For this review, take the finished solid that the model builds, in its own axes (mm). A direction names the side the tool comes from. Round coordinates to 2 decimals unless told otherwise and drop trailing zeros. Order: outer loops, then holes, each group sorted by start corner. A loop starts at its lowest first (then second) coordinate and runs counter-clockwise, first axis right, second up. Notation, with made-up numbers: (49, 26.5) - (62, 26.5) arc R20 cw to (62, 48.5) - close; hole circle Ø5 at (12, -28). An arc over 180 degrees is marked (long way). Write each question's results on one line, items separated by ' | '. Start each with the question number.
(1) Insertion check: pin 1 Ø4 at (x, y) = (4.5, -2.5) entering from +Z; pin 2 Ø4 at (x, y) = (15.5, 3) entering from +Z; pin 3 Ø10.5 at (x, z) = (0, 43.5) entering from +Y; pin 4 Ø6.5 at (y, z) = (-2, 13.5) entering from -X. Each pin has a flat end and moves straight along its axis. Give the tip position at first contact, or say it passes through.
(2) Take a section at C-C, the plane z = 43.5. Give the boundary of the cut face in (x, y).
(3) Take a section at D-D, the plane y = 5.75. Give the boundary of the cut face in (x, z).
(4) For L1, parallel to Z at x = 5.5, y = -0.75; L2, parallel to X at y = -3.5, z = 24.5; L3, parallel to Y at x = -9.4, z = 1.2, list the stretches that pass through material, from the lowest coordinate up. Write a range as from..to.
(5) Draft analysis for pull direction Y (two halves, no side actions). For faces 1 (the cylindrical face through (0, 0, 53)), 2 (the flat face through (0, 6.5, 22)), 3 (the cylindrical face through (8.66, 3.32, 1.97)), state which applies: pulls with the +Y half, pulls with the -Y half, needs draft (parallel to the pull), parting line crosses it, or undercut.
(6) For faces 4 (the flat face through (-3.5, 0, 19)), 5 (the flat face through (13, 0, 4)), 6 (the flat face through (0, 0, 0)), 7 (the cylindrical face through (-6.26, 1.3, 1.97)), 8 (the flat face through (20, 0, 2)), list the 3-axis set-ups (+Z, -Z, +X, -X, +Y, -Y) from which the entire face can be reached by the end or side of a thin tool; tool diameter is ignored.
(7) Take a section at A-A, the plane y = 0. Give the boundary of the cut face in (x, z).
(8) Take a section at B-B, the plane x = 0. Give the boundary of the cut face in (y, z), plus the area to 3 significant figures.
Autodesk Inventor part; units mm, degrees
ref_plane "工作平面3" through (-20, 0, 0) normal (0, 1, 0) x (1, 0, 0)
ref_plane "YZ Plane" through (0, 0, 0) normal (1, 0, 0) x (0, 1, 0)
ref_plane "XZ Plane" through (0, 0, 0) normal (0, 1, 0) x (-1, 0, 0)
sketch "草圖1" plane through (0, 0, 0) normal (0, 0, 1) x (1, 0, 0)
  line L0 (-20, 6.5) -> (20, 6.5)
  line L1 (20, 6.5) -> (20, -6.5)
  line L2 (20, -6.5) -> (-20, -6.5)
  line L3 (-20, -6.5) -> (-20, 6.5)
  line L4 (-20, 6.5) -> (20, -6.5) construction
  line L5 (20, 6.5) -> (-20, -6.5) construction
  circle A0 centre (-9.4, 0) radius 3.4
  circle A1 centre (9.4, 0) radius 3.4
  point P0 (0, 0)
  dimension "d0" = 40
  dimension "d1" = 13
  dimension "d2" = 6.8
  dimension "d3" = 6.8
extrude "擠出1" add sketch "草圖1" along normal blind 4
sketch "草圖3" plane through (0, 0, 4) normal (0, 0, 1) x (1, 0, 0)
  line L0 (3.5, -6.5) -> (-3.5, -6.5)
  line L1 (-3.5, -6.5) -> (-3.5, 6.5)
  line L2 (-3.5, 6.5) -> (3.5, 6.5)
  line L3 (3.5, 6.5) -> (3.5, -6.5)
  line L4 (3.5, -6.5) -> (-3.5, 6.5) construction
  line L5 (-3.5, -6.5) -> (3.5, 6.5) construction
  point P0 (0, 0)
  dimension "d8" = 7
  dimension "d9" = 13
extrude "擠出2" add sketch "草圖3" along normal blind 33
ref_plane "工作平面3" through (-20, 0, 0) normal (0, 1, 0) x (1, 0, 0)
sketch "草圖5" plane through (-20, 0, 0) normal (0, 1, 0) x (1, 0, 0)
  circle A0 centre (20, -43.5) radius 6.5
  circle A1 centre (20, -43.5) radius 9.5
  point P0 (20, 0)
  dimension "d22" = 13
  dimension "d23" = 19
extrude "擠出4" add sketch "草圖5" along normal mid plane 13
properties part number "T字形固定件v2"
Results below:
1) pin 1: stops at z = 52.67 | pin 2: stops at z = 4 | pin 3: passes through | pin 4: stops at x = -3.5
2) outline: (-9.5, -6.5) - (-6.5, -6.5) - (-6.5, 6.5) - (-9.5, 6.5) - close; (6.5, -6.5) - (9.5, -6.5) - (9.5, 6.5) - (6.5, 6.5) - close
3) outline: (-20, 0) - (20, 0) - (20, 4) - (3.5, 4) - (3.5, 34.67) arc R9.5 ccw (long way) to (-3.5, 34.67) - (-3.5, 4) - (-20, 4) - close; hole circle Ø13 at (0, 43.5)
4) L1: z = 0..4, 35.75..40.04, 46.96..51.25 | L2: x = -3.5..3.5 | L3: y = -6.5..-3.4, 3.4..6.5
5) face 1: needs draft | face 2: pulls with the +Y half | face 3: undercut
6) face 4: -X, +Y, -Y | face 5: +X, +Y, -Y | face 6: -Z, +X, -X, +Y, -Y | face 7: -Z | face 8: +Z, -Z, +X, +Y, -Y
7) outline: (-20, 0) - (-12.8, 0) - (-12.8, 4) - (-20, 4) - close; (-6, 0) - (6, 0) - (6, 4) - (3.5, 4) - (3.5, 34.67) arc R9.5 ccw (long way) to (-3.5, 34.67) - (-3.5, 4) - (-6, 4) - close; (12.8, 0) - (20, 0) - (20, 4) - (12.8, 4) - close; hole circle Ø13 at (0, 43.5)
8) outline: (-6.5, 0) - (6.5, 0) - (6.5, 37) - (-6.5, 37) - close; (-6.5, 50) - (6.5, 50) - (6.5, 53) - (-6.5, 53) - close | area: 520 mm^2
